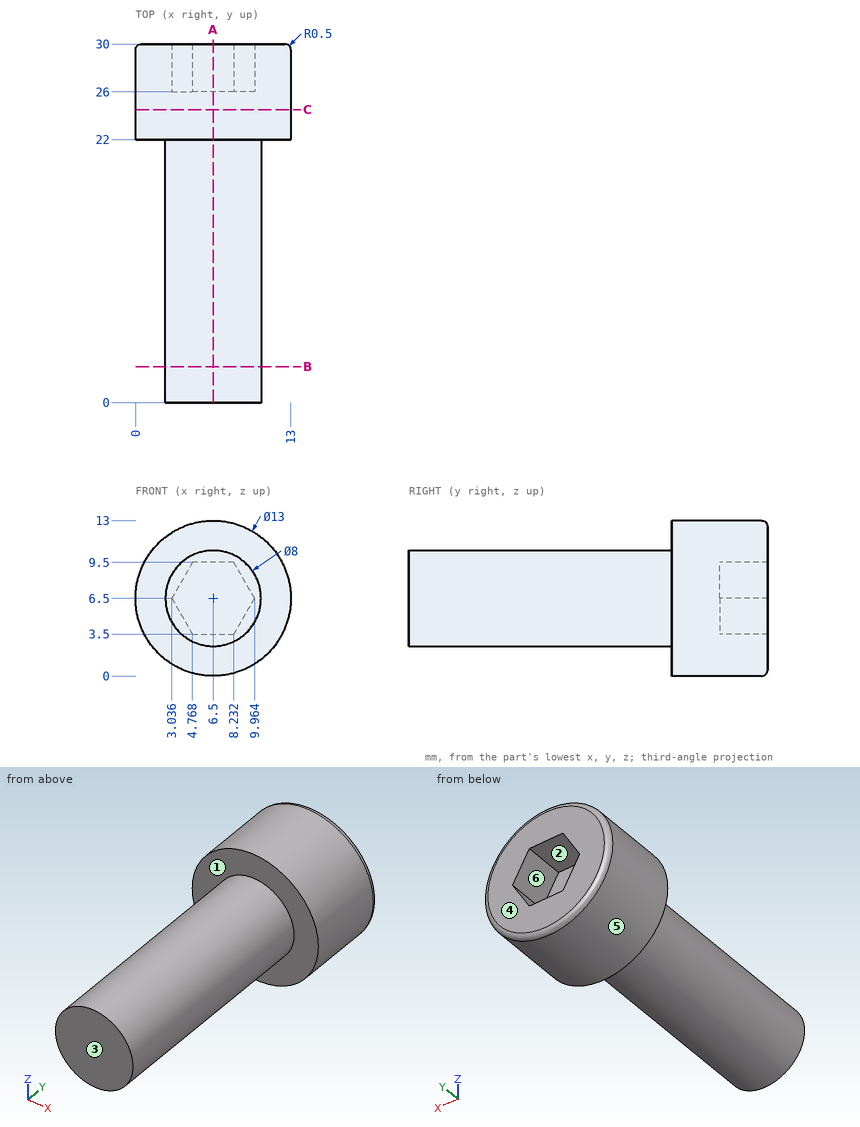
Part print with two shaded views. Sizes in mm from the minimum x, y, z corner. A direction names the side the tool comes from. Coordinates: 2 decimals unless noted, no trailing zeros. Order: outer loops, then holes, each group sorted by start corner. A loop starts at its lowest first (then second) coordinate and runs counter-clockwise, first axis right, second up. Notation, with made-up numbers: (-28, -15.5) - (-17, -15.5) arc R10 cw to (-17, -0.5) - close; hole circle Ø10 at (61, 68). An arc over 180 degrees is marked (long way). Answer in a Markdown table with one row per item.
1. Pull direction Z, two halves, no side cores. Call the marked faces 4, 5 and 6: +Z half, -Z half, draft (parallel to the pull), parting line (faces both ways), or undercut.
Answer:
| item | result |
|---|---|
| face 4 | draft |
| face 5 | parting line |
| face 6 | undercut |
2. Slice it at B-B, the plane y = 3. List the corners of the cut face in (x, z).
Answer:
| item | result |
|---|---|
| outline | circle Ø8 at (6.5, 6.5) |
3. 3-axis set-ups, long thin cutter, end or side, ignore diameter. For the marked faces 1, 2 and 3: which of +Z, -Z, +X, -X, +Y, -Y reach the whole face in a straight line?
Answer:
| item | result |
|---|---|
| face 1 | -Y |
| face 2 | +Y |
| face 3 | +Z, -Z, +X, -X, -Y |
4. Flat gauge pins, fed straight in: P1, Ø5, axis at x = 1.5, y = 4.5, coming from the +Z side; P2, Ø6, axis at y = 16.5, z = 10.5, coming from the -X side; P3, Ø4, axis at x = 9.5, y = 18.5, coming from the -Z side. Where does each tip first touch, or does it go through?
Answer:
| item | result |
|---|---|
| P1 | z = 9.62 |
| P2 | x = 2.63 |
| P3 | z = 2.63 |
5. Slice it at A-A, the plane x = 6.5. List the corners of the cut face in (y, z), then the cut area to 3 significant figures.
Answer:
| item | result |
|---|---|
| outline | (0, 2.5) - (22, 2.5) - (22, 0) - (29.5, 0) arc R0.5 ccw to (30, 0.5) - (30, 3.5) - (26, 3.5) - (26, 9.5) - (30, 9.5) - (30, 12.5) arc R0.5 ccw to (29.5, 13) - (22, 13) - (22, 10.5) - (0, 10.5) - close |
| area | 256 mm² |
6. Drill centre lines: L1, parallel to Y at x = 10.25, z = 2; L2, parallel to Y at x = 4.25, z = 8.5; L3, parallel to Z at x = 4.5, y = 2.75. Where is each one in solid material? Low to high. Write a range as from..to.
Answer:
| item | result |
|---|---|
| L1 | 22..30 |
| L2 | 0..26 |
| L3 | 3.04..9.96 |
7. Slice it at C-C, the plane y = 24.5. List the corners of the cut face in (x, z), then the cut area to 3 significant figures.
Answer:
| item | result |
|---|---|
| outline | circle Ø13 at (6.5, 6.5) |
| area | 133 mm² |
